For this review, take the finished solid that the model builds, in its own axes (mm). A direction names the side the tool comes from. Coordinates: 2 decimals unless noted, no trailing zeros. Loops run counter-clockwise (first coordinate to the right, second up) from the corner with the lowest first, then second, coordinate; pieces in that order, holes last. Notation, with made-up numbers: M 70,85.25 L 94,85.25 A21 cw 94,92.25 Z; hole C 80,5.5 d9. An arc over 180 degrees is marked long. Answer as a JSON object with one key per item and string values. Group by question number.
Item 1: Add section B-B (z = 0). State the section outline as (x, y) points, then the cut area to 4 significant figures.
Item 2: Add section A-A (x = 0). State the section outline as (y, z) points, then the cut area to 4 significant figures.
Item 3: Add section C-C (y = 30). State the section outline as (x, z) points.
Item 4: Add section D-D (z = 9.5). State the section outline as (x, y) points, then the cut area to 3 significant figures.
Item 5: Wall thickness on L1, parallel to Y at x = -3.25, z = -5.75; L2, parallel to X at y = -11, z = 0.5; L3, parallel to X at y = -8, z = 10.25: over which ranges is each line inside the solid? List them lowest first. Write a range as from..to.
Item 6: Insertion check: pin 1 (4 mm diameter, centred on x = 5, z = 8, fed in from -Y); pin 2 (4 mm diameter, centred on y = 19, z = -3, fed in from +X); pin 3 (2 mm diameter, centred on x = 6.5, z = 9, fed in from +Y); pin 4 (1.5 mm diameter, centred on x = 4.5, y = -23.5, fed in from +Z). Each pin has a flat end and moves straight along its axis. Give the tip position at first contact, or say it passes through.
Item 7: Tool access review of faces 1 (the face through (11.923, -9.86, 3.755)), 2 (the face through (-0.54, 43.38, -2.44)), 3 (the face through (-0.54, -29.37, -2.44)): name each direction out of +Z, -Z, +X, -X, +Y, -Y from which nothing blocks a thin tool from reaching the whole face with its end or side.
from build123d import *

# Parameters (mm, degrees)
F0_R     = 2.5
F1_DEPTH = 39
F0_R_2   = 12.5
F2_DEPTH = 20
F3_DEPTH = 88


with BuildPart() as f1:
    # F0 (on Front) → F1 (new body)
    with BuildSketch(Plane.XZ):
        Circle(F0_R)
    extrude(amount=F1_DEPTH)

    # F0 (on Front) → F2 (join)
    with BuildSketch(Plane.XZ):
        Circle(F0_R_2)
        Circle(F0_R, mode=Mode.SUBTRACT)
    extrude(amount=F2_DEPTH)

    # F0 (on Front) → F3 (join)
    with BuildSketch(Plane.XZ):
        Circle(F0_R)
    extrude(amount=-F3_DEPTH)


solid = f1.part
From the geometry:
{
 "1": {"outline": "M -12.5,-20 L -2.5,-20 L -2.5,-39 L 2.5,-39 L 2.5,-20 L 12.5,-20 L 12.5,0 L 2.5,0 L 2.5,88 L -2.5,88 L -2.5,0 L -12.5,0 Z", "area": "1,035 mm²"},
 "2": {"outline": "M -39,-2.5 L -20,-2.5 L -20,-12.5 L 0,-12.5 L 0,-2.5 L 88,-2.5 L 88,2.5 L 0,2.5 L 0,12.5 L -20,12.5 L -20,2.5 L -39,2.5 Z", "area": "1,035 mm²"},
 "3": {"outline": "C 0,0 d5"},
 "4": {"outline": "M -8.12,-20 L 8.12,-20 L 8.12,0 L -8.12,0 Z", "area": "325 mm²"},
 "5": {"L1": "y = -20..0", "L2": "x = -12.49..12.49", "L3": "x = -7.15..7.15"},
 "6": {"pin 1": "stops at y = -20", "pin 2": "stops at x = 2.29", "pin 3": "stops at y = 0", "pin 4": "passes through"},
 "7": {"face 1": "+Y, -Y", "face 2": "+Y", "face 3": "-Y"}
}
